Here's how the part is built. I have some questions about the finished solid (model axes, mm). Round coordinates to 2 decimals unless told otherwise and drop trailing zeros. Order: outer loops, then holes, each group sorted by start corner. A loop starts at its lowest first (then second) coordinate and runs counter-clockwise, first axis right, second up. Notation, with made-up numbers: M 50,4 L 82,4 A16 cw 82,12 Z; hole C 16.5,86 d7. An arc over 180 degrees is marked long. Write each question's results on one line, items separated by ' | '. Start each with the question number.
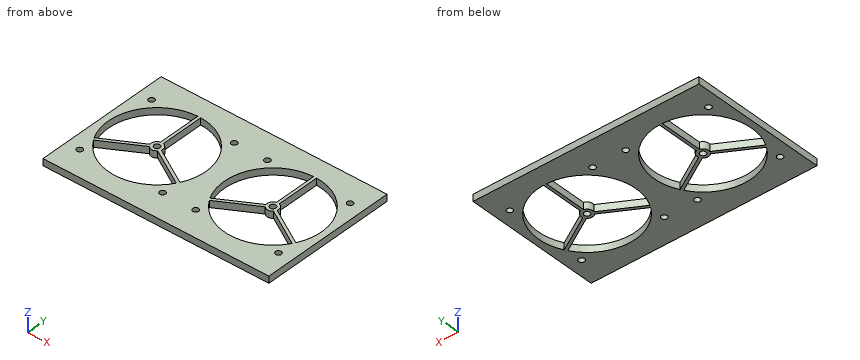
```python
from build123d import *

# Parameters (mm, degrees)
F0_W     = 116
F0_H     = 70
F0_R     = 1.5
F1_DEPTH = 3.5
F2_D     = 3


# Not quite as in the source:
# - a feature names something its author has since deleted; it is built from what else it names


with BuildPart() as f1:
    # F0 (on Top) → F1 (new body)
    with BuildSketch(Plane.XY):
        Rectangle(F0_W, F0_H)
        with BuildLine():
            ThreePointArc((-8.4841098843, -13.1438927866), (-29.75, -25), (-51.0158901157, -13.1438927866))
            Line((-51.0158901157, -13.1438927866), (-31.8905764747, -2.1018878077))
            ThreePointArc((-31.8905764747, -2.1018878077), (-29.75, -3), (-27.6094235253, -2.1018878077))
            Line((-27.6094235253, -2.1018878077), (-8.4841098843, -13.1438927866))
        make_face(mode=Mode.SUBTRACT)
        with BuildLine():
            Line((31.8905764747, -2.1018878077), (51.0158901157, -13.1438927866))
            ThreePointArc((51.0158901157, -13.1438927866), (29.75, -25), (8.4841098843, -13.1438927866))
            Line((8.4841098843, -13.1438927866), (27.6094235253, -2.1018878077))
            ThreePointArc((27.6094235253, -2.1018878077), (29.75, -3), (31.8905764747, -2.1018878077))
        make_face(mode=Mode.SUBTRACT)
        with Locations((-29.75, 0)):
            Circle(F0_R, mode=Mode.SUBTRACT)
        with BuildLine():
            ThreePointArc((-51.7658901157, -11.844854681), (-51.4006350946, 12.5), (-30.5, 24.9887474676))
            Line((-30.5, 24.9887474676), (-30.5, 2.9047375097))
            ThreePointArc((-30.5, 2.9047375097), (-32.3480762114, 1.5), (-32.6405764747, -0.802849702))
            Line((-32.6405764747, -0.802849702), (-51.7658901157, -11.844854681))
        make_face(mode=Mode.SUBTRACT)
        with BuildLine():
            Line((-29, 2.9047375097), (-29, 24.9887474676))
            ThreePointArc((-29, 24.9887474676), (-8.0993649054, 12.5), (-7.7341098843, -11.844854681))
            Line((-7.7341098843, -11.844854681), (-26.8594235253, -0.802849702))
            ThreePointArc((-26.8594235253, -0.802849702), (-27.1519237886, 1.5), (-29, 2.9047375097))
        make_face(mode=Mode.SUBTRACT)
        with BuildLine():
            ThreePointArc((7.7341098843, -11.844854681), (8.0993649054, 12.5), (29, 24.9887474676))
            Line((29, 24.9887474676), (29, 2.9047375097))
            ThreePointArc((29, 2.9047375097), (27.1519237886, 1.5), (26.8594235253, -0.802849702))
            Line((26.8594235253, -0.802849702), (7.7341098843, -11.844854681))
        make_face(mode=Mode.SUBTRACT)
        with Locations((29.75, 0)):
            Circle(F0_R, mode=Mode.SUBTRACT)
        with BuildLine():
            Line((30.5, 2.9047375097), (30.5, 24.9887474676))
            ThreePointArc((30.5, 24.9887474676), (51.4006350946, 12.5), (51.7658901157, -11.844854681))
            Line((51.7658901157, -11.844854681), (32.6405764747, -0.802849702))
            ThreePointArc((32.6405764747, -0.802849702), (32.3480762114, 1.5), (30.5, 2.9047375097))
        make_face(mode=Mode.SUBTRACT)
    extrude(amount=F1_DEPTH)

    # F2 (through all)
    with Locations(Plane(origin=(0, 0, 0), x_dir=(1, 0, 0), z_dir=(0, 0, -1))):
        with Locations((-51, -21.25), (-51, 21.25), (-8.5, 21.25), (-8.5, -21.25), (8.5, -21.25), (8.5, 21.25), (51, 21.25), (51, -21.25)):
            Hole(F2_D / 2)


solid = f1.part
```
(1) Please list where these lines run through material, in increasing order: line 1 (Y direction, x = 29.75, z = 2.55); line 2 (Y direction, x = -27, z = 1.65); line 3 (X direction, y = -15, z = 2.05).
(2) I want a section at A-A on x = 18. Write out the boundary of the cut face in (y, z), and give its area (3 significant figures).
(3) I want a section at B-B on y = 18.5. Write out the boundary of the cut face in (x, z).
(4) I want a section at C-C on y = -21.25. Write out the boundary of the cut face in (x, z).
(5) I want a section at D-D on z = 2.8. Give the number of separate pieces and of enclosed holes in the cut face, and give its area (3 significant figures).
Solutions:
1) line 1: -35 to -25, -3 to -1.5, 1.5 to 35 | line 2: -35 to -24.85, -2.45 to 1.2, 24.85 to 35 | line 3: -58 to -49.75, -9.75 to 9.75, 49.75 to 58
2) outline: M -35,0 L -22.07,0 L -22.07,3.5 L -35,3.5 Z; M -7.65,0 L -5.92,0 L -5.92,3.5 L -7.65,3.5 Z; M 22.07,0 L 35,0 L 35,3.5 L 22.07,3.5 Z | area: 96.6 mm^2
3) outline: M -58,0 L -46.57,0 L -46.57,3.5 L -58,3.5 Z; M -30.5,0 L -29,0 L -29,3.5 L -30.5,3.5 Z; M -12.93,0 L 12.93,0 L 12.93,3.5 L -12.93,3.5 Z; M 29,0 L 30.5,0 L 30.5,3.5 L 29,3.5 Z; M 46.57,0 L 58,0 L 58,3.5 L 46.57,3.5 Z
4) outline: M -58,0 L -52.5,0 L -52.5,3.5 L -58,3.5 Z; M -49.5,0 L -42.92,0 L -42.92,3.5 L -49.5,3.5 Z; M -16.58,0 L -10,0 L -10,3.5 L -16.58,3.5 Z; M -7,0 L 7,0 L 7,3.5 L -7,3.5 Z; M 10,0 L 16.58,0 L 16.58,3.5 L 10,3.5 Z; M 42.92,0 L 49.5,0 L 49.5,3.5 L 42.92,3.5 Z; M 52.5,0 L 58,0 L 58,3.5 L 52.5,3.5 Z
5) separate pieces: 1 | enclosed holes: 16 | area: 4,380 mm^2
